from build123d import *

# Parameters (mm, degrees)
SKETCH1_W           = 210
SKETCH1_H           = 270
BOSS_EXTRUDE1_DEPTH = 6
BOSS_EXTRUDE2_START = -6
SKETCH2_W           = 10
SKETCH2_H           = 182.647861203
SKETCH2_W_2         = 2.953235851
BOSS_EXTRUDE2_DEPTH = 2
SKETCH3_R           = 1.6
CUT_EXTRUDE1_DEPTH  = 30
CUT_EXTRUDE2_DEPTH  = 10
CUT_EXTRUDE3_DEPTH  = 10


with BuildPart() as part:
    # Sketch1 → Boss-Extrude1 (new body)
    with BuildSketch(Plane(origin=(0, 0, 0), x_dir=(1, 0, 0), z_dir=(0, 1, 0))):
        Rectangle(SKETCH1_W, SKETCH1_H)
        with BuildLine():
            Line((-12.932865781, 105.336093738), (-13.182865781, -0.011865408))
            ThreePointArc((-13.182865781, -0.011865408), (-18.19471711, -4.999985921), (-23.182837623, 0.011865408))
            Line((-23.182837623, 0.011865408), (-22.932837623, 105.359824553))
            ThreePointArc((-22.932837623, 105.359824553), (-17.920986294, 110.347945067), (-12.932865781, 105.336093738))
        make_face(mode=Mode.SUBTRACT)
        with BuildLine():
            Line((12.932865781, -105.312362923), (13.182865781, 0.035596223))
            ThreePointArc((13.182865781, 0.035596223), (18.19471711, 5.023716736), (23.182837623, 0.011865408))
            Line((23.182837623, 0.011865408), (22.932837623, -105.336093738))
            ThreePointArc((22.932837623, -105.336093738), (17.920986294, -110.324214252), (12.932865781, -105.312362923))
        make_face(mode=Mode.SUBTRACT)
    extrude(amount=BOSS_EXTRUDE1_DEPTH)

    # Sketch2 → Boss-Extrude2 (add)
    with BuildSketch(Plane(origin=(0, 6, 0), x_dir=(-1, 0, 0), z_dir=(0, 1, 0)).offset(BOSS_EXTRUDE2_START)):
        with Locations((36.432851702, 5.676069398)):
            Rectangle(SKETCH2_W, SKETCH2_H)
        with Locations((24.456233776, 5.676069398)):
            Rectangle(SKETCH2_W_2, SKETCH2_H)
    boss_extrude2 = extrude(amount=-BOSS_EXTRUDE2_DEPTH)

    # Mirror1: Boss-Extrude2 across plane
    add(boss_extrude2.mirror(Plane(origin=(0, 0, 0), x_dir=(0, 0, 1), z_dir=(1, 0, 0))))

    # Sketch3 → Cut-Extrude1 (cut)
    with BuildSketch(Plane.XZ):
        with Locations(Location((-102, 132, 0), (0, 0, 270))):
            Circle(SKETCH3_R)
        with Locations(Location((0, 132, 0), (0, 0, 270))):
            Circle(SKETCH3_R)
        with Locations(Location((102, 132, 0), (0, 0, 270))):
            Circle(SKETCH3_R)
        with Locations(Location((-102, 0, 0), (0, 0, 270))):
            Circle(SKETCH3_R)
        with Locations(Location((-102, -132, 0), (0, 0, 270))):
            Circle(SKETCH3_R)
        with Locations(Location((102, -132, 0), (0, 0, 270))):
            Circle(SKETCH3_R)
        with Locations(Location((102, 0, 0), (0, 0, 270))):
            Circle(SKETCH3_R)
    extrude(amount=-CUT_EXTRUDE1_DEPTH, mode=Mode.SUBTRACT)

    # Sketch4 → Cut-Extrude2 (cut)
    with BuildSketch(Plane.XZ):
        with BuildLine():
            Line((-8.182851702, 5), (-18.182851702, 5))
            Line((-18.182851702, 5), (-18.051918998, -52.673972533))
            Line((-18.051918998, -52.673972533), (-18.182851702, -110.347945067))
            Line((-18.182851702, -110.347945067), (-8.182851702, -110.347945067))
            ThreePointArc((-8.182851702, -110.347945067), (-4.651515343, -108.887671542), (-3.182865781, -105.359810475))
            Line((-3.182865781, -105.359810475), (-3.05783764, -52.673972533))
            Line((-3.05783764, -52.673972533), (-3.182865781, 0.011865408))
            ThreePointArc((-3.182865781, 0.011865408), (-4.651515343, 3.539726475), (-8.182851702, 5))
        make_face()
    extrude(amount=-CUT_EXTRUDE2_DEPTH, mode=Mode.SUBTRACT)

    # Sketch5 → Cut-Extrude3 (cut)
    with BuildSketch(Plane.XZ):
        with BuildLine():
            Line((7.920986294, -5.023730815), (17.920986294, -5.023730815))
            Line((17.920986294, -5.023730815), (17.790053591, 52.650241718))
            Line((17.790053591, 52.650241718), (17.920986294, 110.324214252))
            Line((17.920986294, 110.324214252), (7.920986294, 110.324214252))
            ThreePointArc((7.920986294, 110.324214252), (4.389649935, 108.863940727), (2.921000373, 105.336079659))
            Line((2.921000373, 105.336079659), (2.795972232, 52.650241718))
            Line((2.795972232, 52.650241718), (2.921000373, -0.035596223))
            ThreePointArc((2.921000373, -0.035596223), (4.389649935, -3.56345729), (7.920986294, -5.023730815))
        make_face()
    extrude(amount=-CUT_EXTRUDE3_DEPTH, mode=Mode.SUBTRACT)


solid = part.part
Build history of the part. All positions in model axes, mm. A direction names the side the tool comes from. Coordinates: 2 decimals unless noted, no trailing zeros. Write each loop counter-clockwise with the first axis right and the second up, starting at its lowest first coordinate (ties: lowest second). Pieces come first, ordered by that corner, then holes. Notation, with made-up numbers: (-13.75, 5) -> (14.25, 5) arc R27 cw to (14.25, 35) -> close; hole circle Ø4 at (65.5, 18.5). An arc over 180 degrees is marked (long way). Use CSV: the item, a comma, the result in double quotes. Start each with the question number.
Q1. 3-axis set-ups, long thin cutter, end or side, ignore diameter. For faces 5 (the flat face through (36, -2, 7)), 6 (the flat face through (-13, 3, 5)): which of +Z, -Z, +X, -X, +Y, -Y reach the whole face in a straight line?
Q2. Pull direction X, two halves, no side cores. Call faces 1 (the flat face through (13, 3, -5.024)), 2 (the cylindrical face through (21.587, 2.958, -3.686)), 3 (the flat face through (-1, 3, 135)), 4 (the flat face through (-105, 3, 2)): released by +X, released by -X, zero draft, split by the parting line, or undercut.
Q3. Cut at A-A, the plane y = 3. State how many separate pieces and enclosed holes the cut face has, then the cut area to 3 significant figures.
Q4. Cut at D-D, the plane z = 56. List the corners of the cut face in (x, y), then the cut area to 3 significant figures.
Q5. Drill centre lines: probe 1 along X at (y, z) = (4.55, 0); probe 2 along X at (y, z) = (-1.5, 63); probe 3 along Z at (x, y) = (102, 3.9). Where is each one in solid material? Low to high.
Q6. Cut at C-C, the plane x = -36.5. List the corners of the cut face in (y, z).
Q7. Flat gauge pins, fed straight in: pin 1 Ø1 at (y, z) = (-1.5, -39) entering from -X; pin 2 Ø0.6 at (y, z) = (-1, 24) entering from +X; pin 3 Ø1.5 at (x, z) = (11.5, -42.5) entering from -Y; pin 4 Ø2 at (y, z) = (-0.5, 30.5) entering from +X. Where does each tip first touch, or does it go through?
Q8. Cut at B-B, the plane z = -57. List the corners of the cut face in (x, y), then the cut area to 3 significant figures.
Checked values:
1,face 5,"+Z, -Z, +X, -X, -Y"
1,face 6,"+Y, -Y"
2,face 1,"undercut"
2,face 2,"undercut"
2,face 3,"zero draft"
2,face 4,"released by -X"
3,separate pieces,"1"
3,enclosed holes,"9"
3,area,"52,100 mm²"
4,outline,"(-105, 0) -> (-41.43, 0) -> (-41.43, -2) -> (-31.43, -2) -> (-31.43, 0) -> (-25.93, 0) -> (-25.93, -2) -> (-22.98, -2) -> (-22.98, 0) -> (2.8, 0) -> (2.8, 6) -> (-105, 6) -> close; (22.98, -2) -> (25.93, -2) -> (25.93, 0) -> (31.43, 0) -> (31.43, -2) -> (41.43, -2) -> (41.43, 0) -> (105, 0) -> (105, 6) -> (23.05, 6) -> (23.05, 0) -> (22.98, 0) -> close"
4,area,"1,190 mm²"
5,probe 1,"x = -105 to -103.6, -100.4 to -23.18, -3.18 to 2.92, 23.18 to 100.4, 103.6 to 105"
5,probe 2,"x = -41.43 to -31.43, -25.93 to -22.98, 22.98 to 25.93, 31.43 to 41.43"
5,probe 3,"z = -135 to -133.6, -130.4 to -1.6, 1.6 to 130.4, 133.6 to 135"
6,outline,"(-2, -85.65) -> (0, -85.65) -> (0, -135) -> (6, -135) -> (6, 135) -> (0, 135) -> (0, 97) -> (-2, 97) -> close"
7,pin 1,"stops at x = -41.43"
7,pin 2,"stops at x = 41.43"
7,pin 3,"stops at y = 0"
7,pin 4,"stops at x = 105"
8,outline,"(-105, 0) -> (-41.43, 0) -> (-41.43, -2) -> (-31.43, -2) -> (-31.43, 0) -> (-25.93, 0) -> (-25.93, -2) -> (-22.98, -2) -> (-22.98, 0) -> (-23.05, 0) -> (-23.05, 6) -> (-105, 6) -> close; (-3.07, 0) -> (22.98, 0) -> (22.98, -2) -> (25.93, -2) -> (25.93, 0) -> (31.43, 0) -> (31.43, -2) -> (41.43, -2) -> (41.43, 0) -> (105, 0) -> (105, 6) -> (-3.07, 6) -> close"
8,area,"1,190 mm²"
